Part model, mm, in its own coordinate system. Face numbers are marked on the shaded views. A direction names the side the tool comes from. Coordinates: 2 decimals unless noted, no trailing zeros. Loops run counter-clockwise (first coordinate to the right, second up) from the corner with the lowest first, then second, coordinate; pieces in that order, holes last.
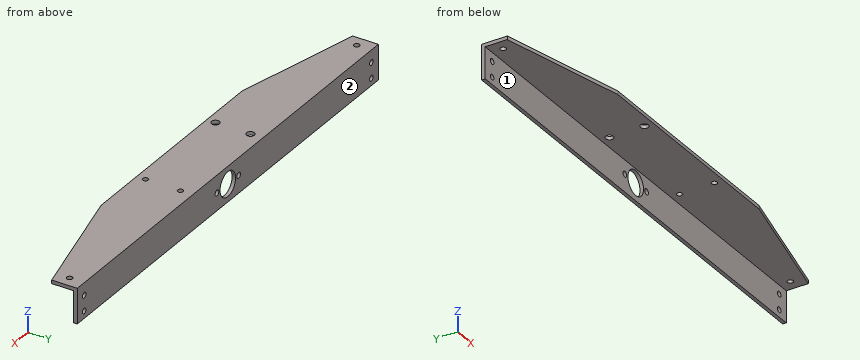
```python
from build123d import *

# Parameters (mm, degrees)
BOSS_EXTRUDE1_DEPTH = 215
SKETCH2_R           = 2.5
SKETCH2_R_2         = 3.57
CUT_EXTRUDE1_DEPTH  = 4.175
CUT_EXTRUDE2_DEPTH  = 3.175
SKETCH4_R           = 2.5
CUT_EXTRUDE3_DEPTH  = 3.175
CUT_EXTRUDE4_REACH  = 5.175
SKETCH5_R           = 11.1125
SKETCH6_R           = 2.6
CUT_EXTRUDE5_DEPTH  = 3.175
SKETCH7_R           = 2.6
CUT_EXTRUDE6_DEPTH  = 3.175


with BuildPart() as part:
    # Sketch1 → Boss-Extrude1 (new body, symmetric)
    with BuildSketch(Plane(origin=(0, 0, 0), x_dir=(0, 0, -1), z_dir=(1, 0, 0))):
        Polygon((0, 0), (31.75, 0), (31.75, -3.175), (3.175, -3.175), (3.175, -50.8), (0, -50.8), align=None)
    extrude(amount=BOSS_EXTRUDE1_DEPTH, both=True)

    # Sketch2 → Cut-Extrude1 (cut, through all)
    with BuildSketch(Plane(origin=(0, 0, -3.175), x_dir=(-1, 0, 0), z_dir=(0, 0, -1))):
        with Locations((-50, -11.175)):
            Circle(SKETCH2_R)
        with Locations((50, -11.175)):
            Circle(SKETCH2_R_2)
        with Locations((50, -42.8)):
            Circle(SKETCH2_R_2)
        with Locations((-50, -42.8)):
            Circle(SKETCH2_R)
    extrude(amount=-CUT_EXTRUDE1_DEPTH, mode=Mode.SUBTRACT)

    # Sketch3 → Cut-Extrude2 (cut)
    with BuildSketch(Plane(origin=(0, 0, -3.175), x_dir=(-1, 0, 0), z_dir=(0, 0, -1))):
        Polygon((215, -50.8), (100.7, -50.8), (215, -23.175), align=None)
        Polygon((-215, -23.175), (-215, -50.8), (-100.7, -50.8), align=None)
    extrude(amount=-CUT_EXTRUDE2_DEPTH, mode=Mode.SUBTRACT)

    # Sketch4 → Cut-Extrude3 (cut)
    with BuildSketch(Plane(origin=(0, 0, 0), x_dir=(1, 0, 0), z_dir=(0, 1, 0))):
        with Locations((-205, 11.176)):
            Circle(SKETCH4_R)
        with Locations((-205, 25.176)):
            Circle(SKETCH4_R)
        with Locations((205, 25.176)):
            Circle(SKETCH4_R)
        with Locations((205, 11.176)):
            Circle(SKETCH4_R)
    extrude(amount=-CUT_EXTRUDE3_DEPTH, mode=Mode.SUBTRACT)

    # Sketch5 → Cut-Extrude4 (cut, up to next)
    with BuildSketch(Plane.XZ.offset(3.175), mode=Mode.PRIVATE) as cut_extrude4_sk1:
        with Locations((0, -15.875)):
            Circle(SKETCH5_R)
    cut_extrude4_tool1 = extrude(cut_extrude4_sk1.sketch, amount=-CUT_EXTRUDE4_REACH, mode=Mode.PRIVATE) & part.part
    add(cut_extrude4_tool1.solids().sort_by_distance((0, -3.175, -15.875))[0], mode=Mode.SUBTRACT)

    # Sketch6 → Cut-Extrude5 (cut)
    with BuildSketch(Plane.XY):
        with Locations((205, -13.175000066)):
            Circle(SKETCH6_R)
        with Locations((-205, -13.175000066)):
            Circle(SKETCH6_R)
    extrude(amount=-CUT_EXTRUDE5_DEPTH, mode=Mode.SUBTRACT)

    # Sketch7 → Cut-Extrude6 (cut)
    with BuildSketch(Plane(origin=(0, 0, 0), x_dir=(1, 0, 0), z_dir=(0, 1, 0))):
        with Locations((15.5, 15.875)):
            Circle(SKETCH7_R)
        with Locations((-15.5, 15.875)):
            Circle(SKETCH7_R)
    extrude(amount=-CUT_EXTRUDE6_DEPTH, mode=Mode.SUBTRACT)


solid = part.part
```
Q1. Saw through at D-D (x = 162.5). List the corners of the cut face in (y, z) (3 decimals), plus the area to 3 significant figures.
Q2. Saw through at C-C (x = 66). List the corners of the cut face in (y, z) (3 decimals), plus the area to 3 significant figures.
Q3. Drop flat-ended pins along their axis: P1, Ø6, axis at x = 205, z = -25.176, coming from the -Y side (3 decimals); P2, Ø6, axis at x = 87.5, y = -24.5, coming from the -Z side (3 decimals). Give the stop position or say it passes through.
Q4. Probe line 1 (Z direction, x = 205, y = -2.4); line 2 (Z direction, x = 76.5, y = -15) (3 decimals). List the from-to ranges inside material, lowest first.
Q5. Tool access for the marked faces 1 and 2: list every direction of +Z, -Z, +X, -X, +Y, -Y with a clear straight run to the whole face (end or side of a thin tool).
Q6. Saw through at B-B (x = -50). List the corners of the cut face in (y, z) (3 decimals), plus the area to 3 significant figures.
Checked values:
1. outline: (-35.864, -3.175) - (-3.175, -3.175) - (-3.175, -31.75) - (0, -31.75) - (0, 0) - (-35.864, 0) - close
1. area: 205 mm2
2. outline: (-50.8, -3.175) - (-3.175, -3.175) - (-3.175, -31.75) - (0, -31.75) - (0, 0) - (-50.8, 0) - close
2. area: 252 mm2
3. P1: stops at y = -3.175
3. P2: stops at z = -3.175
4. line 1: z = -31.75 to -27.68, -22.68 to -13.68, -8.68 to 0
4. line 2: z = -3.175 to 0
5. face 1: -Z, +X, -X, -Y
5. face 2: +Z, -Z, +X, -X, +Y
6. outline: (-50.8, -3.175) - (-46.37, -3.175) - (-46.37, 0) - (-50.8, 0) - close; (-39.23, -3.175) - (-14.745, -3.175) - (-14.745, 0) - (-39.23, 0) - close; (-7.605, -3.175) - (-3.175, -3.175) - (-3.175, -31.75) - (0, -31.75) - (0, 0) - (-7.605, 0) - close
6. area: 207 mm2
